Autodesk Inventor part; units mm, degrees
ref_plane "YZ Plane" through (0, 0, 0) normal (1, 0, 0) x (0, 1, 0)
ref_plane "XZ Plane" through (0, 0, 0) normal (0, 1, 0) x (-1, 0, 0)
ref_plane "XY Plane" through (0, 0, 0) normal (0, 0, 1) x (1, 0, 0)
sketch "Sketch1" plane through (0, 0, 0) normal (0, 0, 1) x (1, 0, 0)
  arc A0 (127, -140) -> (122, -135) centre (122, -140) ccw
  line L0 (122, -135) -> (119.8284, -135)
  line L1 (119.8284, -135) -> (119.8284, -145)
  line L2 (119.8284, -145) -> (114.1716, -145)
  line L3 (114.1716, -145) -> (114.1716, -135)
  line L4 (114.1716, -135) -> (109.5, -135)
  arc A1 (107, -132.5) -> (109.5, -135) centre (109.5, -132.5) ccw
  line L5 (107, -132.5) -> (107, 132.5)
  arc A2 (109.5, 135) -> (107, 132.5) centre (109.5, 132.5) ccw
  line L6 (109.5, 135) -> (114.1716, 135)
  line L7 (114.1716, 135) -> (114.1716, 145)
  line L8 (114.1716, 145) -> (119.8284, 145)
  line L9 (119.8284, 145) -> (119.8284, 135)
  line L10 (119.8284, 135) -> (122, 135)
  arc A3 (122, 135) -> (127, 140) centre (122, 140) ccw
  line L11 (127, 140) -> (127, 165)
  arc A4 (127, 165) -> (122, 170) centre (122, 165) ccw
  line L12 (122, 170) -> (-122, 170)
  arc A5 (-122, 170) -> (-127, 165) centre (-122, 165) ccw
  line L13 (-127, 165) -> (-127, 140)
  arc A6 (-127, 140) -> (-122, 135) centre (-122, 140) ccw
  line L14 (-122, 135) -> (-119.8284, 135)
  line L15 (-119.8284, 135) -> (-119.8284, 145)
  line L16 (-119.8284, 145) -> (-114.1716, 145)
  line L17 (-114.1716, 145) -> (-114.1716, 135)
  line L18 (-114.1716, 135) -> (-109.5, 135)
  arc A7 (-107, 132.5) -> (-109.5, 135) centre (-109.5, 132.5) ccw
  line L19 (-107, 132.5) -> (-107, -132.5)
  arc A8 (-109.5, -135) -> (-107, -132.5) centre (-109.5, -132.5) ccw
  line L20 (-109.5, -135) -> (-114.1716, -135)
  line L21 (-114.1716, -135) -> (-114.1716, -145)
  line L22 (-114.1716, -145) -> (-119.8284, -145)
  line L23 (-119.8284, -145) -> (-119.8284, -135)
  line L24 (-119.8284, -135) -> (-122, -135)
  arc A9 (-122, -135) -> (-127, -140) centre (-122, -140) ccw
  line L25 (-127, -140) -> (-127, -165)
  arc A10 (-127, -165) -> (-122, -170) centre (-122, -165) ccw
  line L26 (-122, -170) -> (122, -170)
  arc A11 (122, -170) -> (127, -165) centre (122, -165) ccw
  line L27 (127, -165) -> (127, -140)
  line L28 (113, -142) -> (112, -142)
  line L29 (112, -142) -> (112, -138)
  line L30 (112, -138) -> (113, -138)
  line L31 (113, -138) -> (113, -142)
  line L32 (121, -142) -> (121, -138)
  line L33 (121, -138) -> (122, -138)
  line L34 (122, -138) -> (122, -142)
  line L35 (122, -142) -> (121, -142)
  line L36 (-112, -142) -> (-113, -142)
  line L37 (-113, -142) -> (-113, -138)
  line L38 (-113, -138) -> (-112, -138)
  line L39 (-112, -138) -> (-112, -142)
  line L40 (-121, -138) -> (-121, -142)
  line L41 (-121, -142) -> (-122, -142)
  line L42 (-122, -142) -> (-122, -138)
  line L43 (-122, -138) -> (-121, -138)
  line L44 (112, 142) -> (113, 142)
  line L45 (113, 142) -> (113, 138)
  line L46 (113, 138) -> (112, 138)
  line L47 (112, 138) -> (112, 142)
  line L48 (121, 138) -> (121, 142)
  line L49 (121, 142) -> (122, 142)
  line L50 (122, 142) -> (122, 138)
  line L51 (122, 138) -> (121, 138)
  line L52 (-122, 138) -> (-122, 142)
  line L53 (-122, 142) -> (-121, 142)
  line L54 (-121, 142) -> (-121, 138)
  line L55 (-121, 138) -> (-122, 138)
  line L56 (-112, 142) -> (-112, 138)
  line L57 (-112, 138) -> (-113, 138)
  line L58 (-113, 138) -> (-113, 142)
  line L59 (-113, 142) -> (-112, 142)
  line L60 (-127, 140) -> (-127, -140)
  line L61 (127, -140) -> (127, 140)
  arc A12 (20.5, 83.5) -> (-1.5, 83.5) centre (9.5, 83.5) ccw
  line L62 (20.5, 83.5) -> (20.5, -116.5)
  arc A13 (-1.5, -116.5) -> (20.5, -116.5) centre (9.5, -116.5) ccw
  line L63 (-1.5, -116.5) -> (-1.5, 83.5)
  line L64 (42, -96.4) -> (77, -96.4)
  line L65 (77, -96.4) -> (77, -138.4)
  line L66 (77, -138.4) -> (42, -138.4)
  line L67 (42, -138.4) -> (42, -96.4)
  line L68 (77, 117.6) -> (42, 117.6)
  line L69 (42, 117.6) -> (42, 159.6)
  line L70 (42, 159.6) -> (77, 159.6)
  line L71 (77, 159.6) -> (77, 117.6)
  line L72 (-77, -96.4) -> (-42, -96.4)
  line L73 (-42, -96.4) -> (-42, -138.4)
  line L74 (-42, -138.4) -> (-77, -138.4)
  line L75 (-77, -138.4) -> (-77, -96.4)
  line L76 (-42, 117.6) -> (-77, 117.6)
  line L77 (-77, 117.6) -> (-77, 159.6)
  line L78 (-77, 159.6) -> (-42, 159.6)
  line L79 (-42, 159.6) -> (-42, 117.6)
  circle A14 centre (0, 165) radius 1.25
  circle A15 centre (0, -165) radius 1.25
  circle A16 centre (-23, -162.38) radius 3.175
  circle A17 centre (-30.6332, -154.7468) radius 0.5
  circle A18 centre (-15.3668, -154.7468) radius 0.5
  point P0 (0, 0)
extrude "Extrusion1" add sketch "Sketch1" along normal blind 6.477 contours L27 A11 L26 A10 L25 A9 L24 L23 L22 L21 L20 A8 L19 A7 L18 L17 L16 L15 L14 A6 L13 A5 L12 A4 L11 A3 L10 L9 L8 L7 L6 A2 L5 A1 L4 L3 L2 L1 L0 A0 | A0 L0 L1 L2 L3 L4 A1 L5 A2 L6 L7 L8 L9 L10 A3 L61 | L60 A6 L14 L15 L16 L17 L18 A7 L19 A8 L20 L21 L22 L23 L24 A9 | L62 A13 L63 A12 | L64 L65 L66 L67 | L68 L69 L70 L71 | L72 L73 L74 L75 | L76 L77 L78 L79 | A14 | A15 | A16 | A17 | A18
sketch "Sketch2" plane through (0, 0, 6.477) normal (0, 0, 1) x (1, 0, 0)
  line L0 (-122, -170) -> (122, -170)
  line L1 (-101.6, 112.2) -> (101.6, 112.2)
  line L2 (101.6, 112.2) -> (101.6, -91)
  line L3 (101.6, -91) -> (-101.6, -91)
  line L4 (-101.6, -91) -> (-101.6, 112.2)
  point P0 (0, 0)
  point P1 (0, -91)
  dimension "d2" = 203.2
  dimension "d4" = 79
extrude "Extrusion2" cut sketch "Sketch2" against normal through all
sketch "Sketch3" plane through (0, 0, 6.477) normal (0, 0, 1) x (1, 0, 0)
  line L0 (-127, 165) -> (-127, -165)
  line L1 (127, 137.6) -> (-127, 137.6)
  line L2 (-127, -116.4) -> (127, -116.4)
  line L3 (-77, -116.4) -> (-42, -116.4)
  line L4 (-42, -116.4) -> (-42, -138.4)
  line L5 (-42, -138.4) -> (-77, -138.4)
  line L6 (-77, -138.4) -> (-77, -116.4)
  line L7 (77, -116.4) -> (42, -116.4)
  line L8 (42, -116.4) -> (42, -138.4)
  line L9 (42, -138.4) -> (77, -138.4)
  line L10 (77, -138.4) -> (77, -116.4)
  line L11 (-77, 137.6) -> (-42, 137.6)
  line L12 (-42, 137.6) -> (-42, 159.6)
  line L13 (-42, 159.6) -> (-77, 159.6)
  line L14 (-77, 159.6) -> (-77, 137.6)
  line L15 (77, 137.6) -> (42, 137.6)
  line L16 (42, 137.6) -> (42, 159.6)
  line L17 (42, 159.6) -> (77, 159.6)
  line L18 (77, 159.6) -> (77, 137.6)
  line L19 (-42, -138.4) -> (42, -138.4)
  line L20 (-42, 159.6) -> (42, 159.6)
  point P0 (0, 0)
  point P1 (0, -138.4)
  point P2 (0, -116.4)
  point P3 (0, 159.6)
  dimension "d7" = 22
  dimension "d9" = 35
  dimension "d10" = 50
extrude "Extrusion3" cut sketch "Sketch3" against normal through all contours L2 L4 L5 L6 | L14 L13 L12 L1 | L16 L17 L18 L1 | L2 L10 L9 L8
sketch "Sketch4" plane through (0, 0, 6.477) normal (0, 0, 1) x (1, 0, 0)
  circle A0 centre (0, 165) radius 1.25
  circle A1 centre (0, -165) radius 1.25
  point P0 (0, 0)
extrude "Extrusion4" cut sketch "Sketch4" against normal through all
sketch "Sketch5" plane through (0, 0, 6.477) normal (0, 0, 1) x (1, 0, 0)
  circle A0 centre (-23, -162.38) radius 5.08
  point P0 (0, 0)
extrude "Extrusion5" cut sketch "Sketch5" against normal through all
sketch "Sketch6" plane through (0, 0, 6.477) normal (0, 0, 1) x (1, 0, 0)
  circle A0 centre (-30.6332, -154.7468) radius 0.5
  circle A1 centre (-15.3668, -154.7468) radius 0.5
  circle A2 centre (-23, -162.38) radius 5.08
  line L0 (-15.5, -150) -> (-30.5, -150)
  line L1 (-35.5, -155) -> (-35.5, -165)
  line L2 (-30.5, -170) -> (-15.5, -170)
  line L3 (-10.5, -165) -> (-10.5, -155)
  arc A3 (-30.5, -150) -> (-35.5, -155) centre (-30.5, -155) ccw
  arc A4 (-35.5, -165) -> (-30.5, -170) centre (-30.5, -165) ccw
  arc A5 (-15.5, -170) -> (-10.5, -165) centre (-15.5, -165) ccw
  arc A6 (-10.5, -155) -> (-15.5, -150) centre (-15.5, -155) ccw
  point P0 (0, 0)
extrude "Extrusion6" cut sketch "Sketch6" against normal through all contours A0 | A1
sketch "Sketch7" plane through (0, 0, 6.477) normal (0, 0, 1) x (1, 0, 0)
  line L0 (-101.6, 112.2) -> (101.6, 112.2)
  line L1 (4.7625, 112.2) -> (-4.7625, 112.2)
  line L2 (-4.7625, 112.2) -> (-4.7625, 150.3)
  line L3 (-4.7625, 150.3) -> (4.7625, 150.3)
  line L4 (4.7625, 150.3) -> (4.7625, 112.2)
  point P0 (0, 0)
  point P1 (0, 150.3)
  point P2 (0, 112.2)
  dimension "d19" = 38.1
  dimension "d21" = 9.525
extrude "Extrusion7" cut sketch "Sketch7" against normal through all
fillet "Fillet1" radius 4.7625 4 edges at (4.7625, 112.2, 3.2385) (-4.7625, 112.2, 3.2385) (-4.7625, 150.3, 3.2385) (4.7625, 150.3, 3.2385)
properties part number "BED HOT BED INSET"
Geometry: final body of the model. Coordinates: model frame, mm. A direction names the side the tool comes from. Round coordinates to 2 decimals unless told otherwise and drop trailing zeros. Order: outer loops, then holes, each group sorted by start corner. A loop starts at its lowest first (then second) coordinate and runs counter-clockwise, first axis right, second up. Notation, with made-up numbers: (-25, -13.5) - (33, -13.5) arc R26 ccw to (33, 11.5) - close; hole circle Ø9 at (76.25, 22). An arc over 180 degrees is marked (long way). Write each question's results on one line, items separated by ' | '.
Item 1: Section A-A, the plane x = -92.5. Return the cut outline in (y, z), and give its area (3 significant figures).
Completed:
outline: (-170, 0) - (-91, 0) - (-91, 6.48) - (-170, 6.48) - close; (112.2, 0) - (170, 0) - (170, 6.48) - (112.2, 6.48) - close | area: 886 mm^2
Item 2: Section C-C, the plane x = -23. Return the cut outline in (y, z).
Completed:
outline: (-170, 0) - (-167.46, 0) - (-167.46, 6.48) - (-170, 6.48) - close; (-157.3, 0) - (-91, 0) - (-91, 6.48) - (-157.3, 6.48) - close; (112.2, 0) - (170, 0) - (170, 6.48) - (112.2, 6.48) - close
Item 3: Material intervals for line 1 along Y through (x, z) = (76, 4.75); line 2 along Y through (x, z) = (0, 3); line 3 along X through (y, z) = (40, 2.25), sorted ascending. Write a range as [from, to].
Completed:
line 1: [-170, -138.4], [-116.4, -91], [112.2, 137.6], [159.6, 170] | line 2: [-170, -166.25], [-163.75, -91], [150.3, 163.75], [166.25, 170] | line 3: [-127, -101.6], [101.6, 127]
Item 4: Section B-B, the plane y = 64.5. Return the cut outline in (x, z).
Completed:
outline: (-127, 0) - (-101.6, 0) - (-101.6, 6.48) - (-127, 6.48) - close; (101.6, 0) - (127, 0) - (127, 6.48) - (101.6, 6.48) - close
Item 5: Mould query, pull axis Y, two halves, no side actions, for faces 3 (the flat face through (-2, -111, 6.477)), 4 (the flat face through (2, 170, 3)), 5 (the flat face through (-59, 159.6, 3)). Classes: pulls with the +Y half, pulls with the -Y half, needs draft (parallel to the pull), parting line crosses it, or undercut.
Completed:
face 3: needs draft | face 4: pulls with the +Y half | face 5: undercut
Item 6: Section D-D, the plane z = 4. State how many separate pieces and enclosed holes the cut face has, and give its area (3 significant figures).
Completed:
separate pieces: 1 | enclosed holes: 18 | area: 41,500 mm^2
Item 7: Reachability of faces 1 (the flat face through (-2, -170, 3)), 2 (the flat face through (-42, 148, 3)) from +Z, -Z, +X, -X, +Y, -Y: full face, straight path, thin tool, end or side. Return the list, or none.
Completed:
face 1: +Z, -Z, +X, -X, -Y | face 2: +Z, -Z
